Design review of the part shown in the three views and the two pictorial views. Dimensions are in mm from the part's minimum x, y and z. Round coordinates to 2 decimals unless told otherwise and drop trailing zeros. Loops run counter-clockwise (first coordinate to the right, second up) from the corner with the lowest first, then second, coordinate; pieces in that order, holes last. Notation, with made-up numbers: (57, -35.5) -> (64, -35.5) arc R30 ccw to (64, 3.5) -> close; hole circle Ø8 at (27.25, 24). An arc over 180 degrees is marked (long way). Use a Markdown table: item, result. Add a question column.
1) Insertion check: pin 1 (4 mm diameter, centred on x = 11.47, y = 14.58, fed in from -Z); pin 2 (1.5 mm diameter, centred on y = 5.5, z = 2.5, fed in from +X) (1 decimal); pin 3 (2 mm diameter, centred on x = 6, y = 8, fed in from -Z). Each pin has a flat end and moves straight along its axis. Give the tip position at first contact, or say it passes through.
2) Consider section B-B on z = 1.2. State how many separate pieces and enclosed holes the cut face has, plus the area to 3 significant figures.
3) Consider section D-D on x = 8.5. Give the boundary of the cut face in (y, z).
4) Mouldability with a two-part tool opening along Y and no side actions: class the marked faces 1, 2 and 3 as released by +Y, released by -Y, zero draft, split by the parting line, or undercut.
5) Consider section C-C on y = 6.25. Give the boundary of the cut face in (x, z), plus the area to 3 significant figures.
6) Wall thickness on probe 1 along X at (y, z) = (14.75, 1.6); probe 2 along Y at (x, z) = (12.75, 1.9) (1 decimal); probe 3 along X at (y, z) = (18.75, 0.75) (1 decimal): over which ranges is each line inside the solid? List them lowest first.
7) Consider section A-A on x = 11. Give the boundary of the cut face in (y, z).
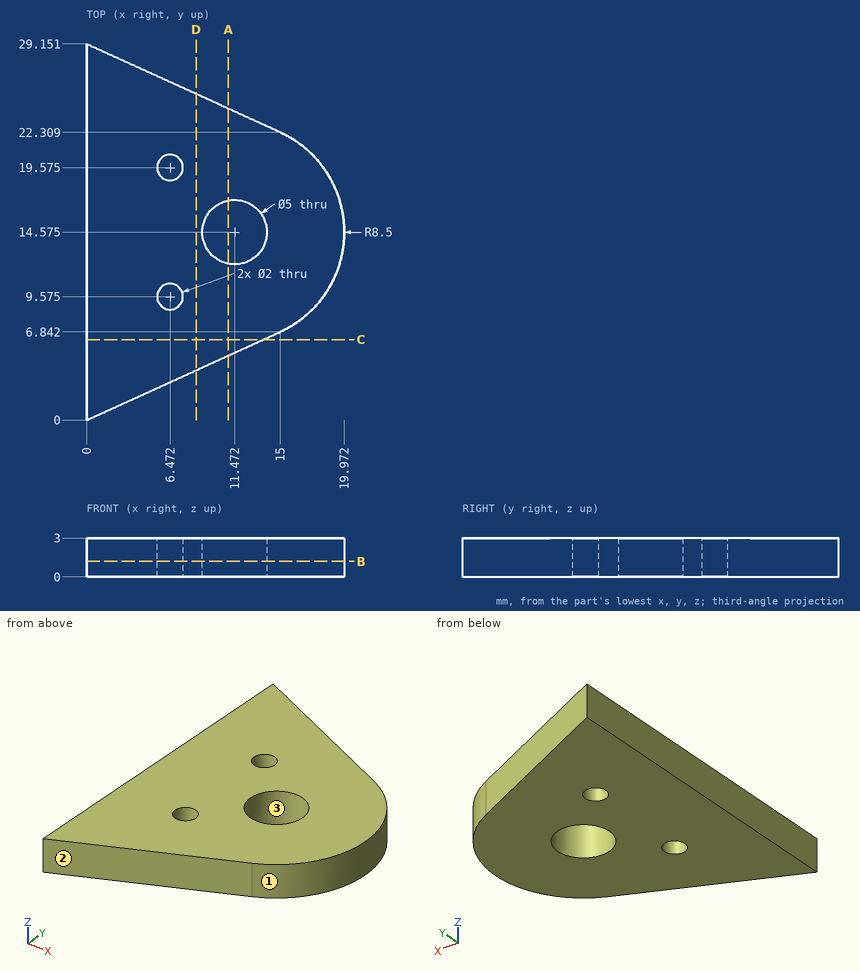
Result set:
| question | item | result |
|---|---|---|
| 1 | pin 1 | through |
| 1 | pin 2 | x = 13.7 |
| 1 | pin 3 | z = 0 |
| 2 | separate pieces | 1 |
| 2 | enclosed holes | 3 |
| 2 | area | 364 mm2 |
| 3 | outline | (3.88, 0) -> (25.27, 0) -> (25.27, 3) -> (3.88, 3) -> close |
| 4 | face 1 | split by the parting line |
| 4 | face 2 | released by -Y |
| 4 | face 3 | undercut |
| 5 | outline | (0, 0) -> (13.7, 0) -> (13.7, 3) -> (0, 3) -> close |
| 5 | area | 41.1 mm2 |
| 6 | probe 1 | 0 to 8.98, 13.97 to 19.97 |
| 6 | probe 2 | 5.8 to 12.4, 16.7 to 23.3 |
| 6 | probe 3 | 0 to 5.9, 7 to 18.9 |
| 7 | outline | (5.02, 0) -> (12.12, 0) -> (12.12, 3) -> (5.02, 3) -> close; (17.03, 0) -> (24.13, 0) -> (24.13, 3) -> (17.03, 3) -> close |
